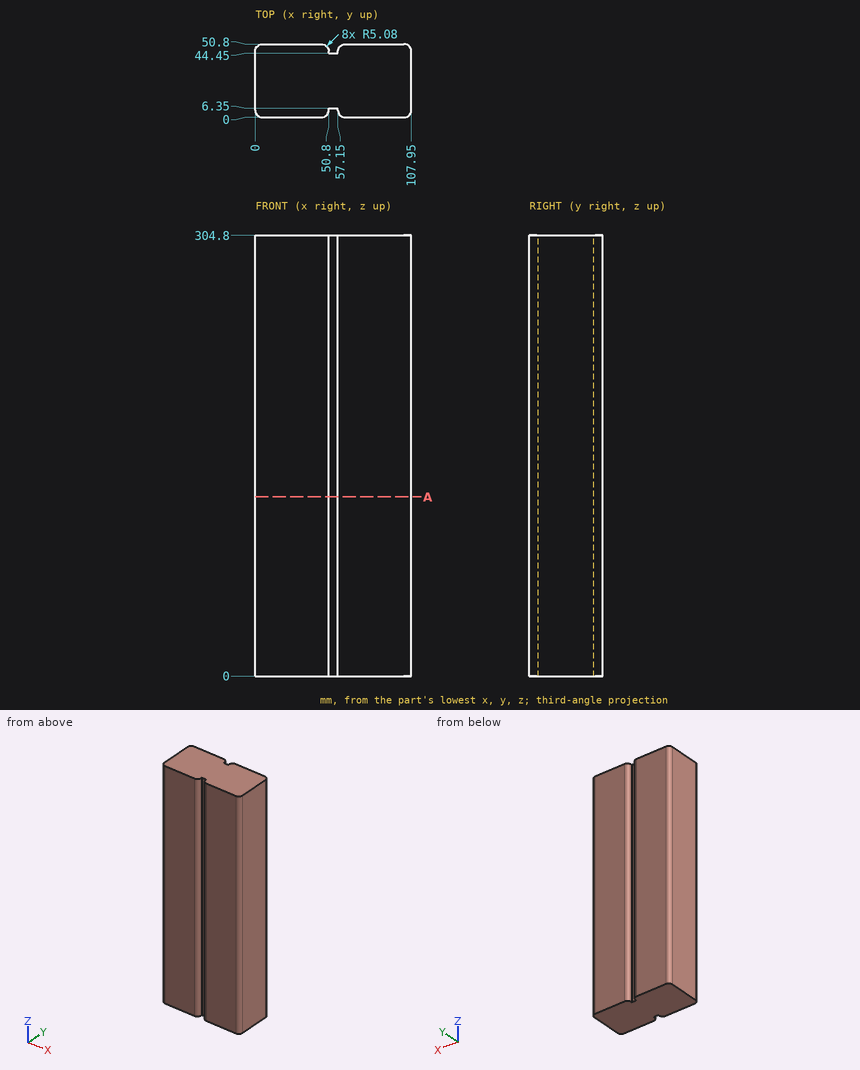
The figure shows three views and two pictorial views of one solid part (mm, origin at its lowest corner). Answer the questions. Give positions to 0.01 mm unless a question says otherwise; leave off trailing zeros. Loops run counter-clockwise (first coordinate to the right, second up) from the corner with the lowest first, then second, coordinate; pieces in that order, holes last. Notation, with made-up numbers: (-40, 33.25) -> (-35, 33.25) arc R30 cw to (-35, 69.25) -> close; hole circle Ø1 at (73.5, 57.5). An arc over 180 degrees is marked (long way). Use a Markdown table: item, result. Add a question column.
1. Find the intervals of material crossed by probe 1 along X at (y, z) = (45, 83.5); probe 2 along Y at (x, z) = (52, 203); probe 3 along Y at (x, z) = (5, 123), in increasing order.
2. Section A-A on z = 124 is taken. Determine the outline of the cut face in (x, y).
3. Flat-ended cylindrical pins translate along their axes: pin 1 Ø1.9 at (x, z) = (53.5, 76.5) entering from +Y; pin 2 Ø3 at (x, z) = (53, 188) entering from -Y. Find the tip coordinate at first contact, or state that the pin passes through.
Results below:
| question | item | result |
|---|---|---|
| 1 | probe 1 | x = 0 to 50.8, 57.15 to 107.95 |
| 1 | probe 2 | y = 6.35 to 44.45 |
| 1 | probe 3 | y = 0 to 50.8 |
| 2 | outline | (0, 5.08) arc R5.08 ccw to (5.08, 0) -> (45.72, 0) arc R5.08 ccw to (50.8, 5.08) -> (50.8, 6.35) -> (57.15, 6.35) -> (57.15, 5.08) arc R5.08 ccw to (62.23, 0) -> (102.87, 0) arc R5.08 ccw to (107.95, 5.08) -> (107.95, 45.72) arc R5.08 ccw to (102.87, 50.8) -> (62.23, 50.8) arc R5.08 ccw to (57.15, 45.72) -> (57.15, 44.45) -> (50.8, 44.45) -> (50.8, 45.72) arc R5.08 ccw to (45.72, 50.8) -> (5.08, 50.8) arc R5.08 ccw to (0, 45.72) -> close |
| 3 | pin 1 | stops at y = 44.45 |
| 3 | pin 2 | stops at y = 6.35 |
